```python
from build123d import *

# Parameters (mm, degrees)
F0_R     = 14.2875
F1_DEPTH = 14.2875
F2_R     = 6.35
F3_DEPTH = 44.45
F4_R     = 4.445
F5_DEPTH = 76.2


with BuildPart() as f1:
    # F0 (on Top) → F1 (new body, symmetric)
    with BuildSketch(Plane.XY):
        Circle(F0_R)
    extrude(amount=F1_DEPTH, both=True)

    # F2 (on face) → F3 (join)
    with BuildSketch(Plane(origin=(0, 0, -14.2875), x_dir=(1, 0, 0), z_dir=(0, 0, -1))):
        Circle(F2_R)
    extrude(amount=F3_DEPTH)

    # F4 (on Right) → F5 (join, symmetric)
    with BuildSketch(Plane.YZ):
        Circle(F4_R)
    extrude(amount=F5_DEPTH, both=True)

    # F6 (on Front) → F7 (revolve)
    with BuildSketch(Plane.XZ):
        with BuildLine():
            Line((-86.36, 0), (-66.04, 0))
            ThreePointArc((-66.04, 0), (-76.2, 10.16), (-86.36, 0))
        make_face()
    revolve(axis=Axis((-76.2, 0, 0), (1, 0, 0)))

    # F8 (on Front) → F9 (revolve)
    with BuildSketch(Plane.XZ):
        with BuildLine():
            Line((66.04, 0), (86.36, 0))
            ThreePointArc((86.36, 0), (76.2, 10.16), (66.04, 0))
        make_face()
    revolve(axis=Axis((76.2, 0, 0), (1, 0, 0)))


solid = f1.part
```
Model file for the job. Use its own axes, mm. A direction names the side the tool comes from. Give positions to 0.01 mm unless a question says otherwise; leave off trailing zeros. Write each loop counter-clockwise with the first axis right and the second up, starting at its lowest first coordinate (ties: lowest second). Pieces come first, ordered by that corner, then holes. Notation, with made-up numbers: (-35.5, 10.5) -> (16.5, 10.5) arc R21 ccw to (16.5, 33.5) -> close; hole circle Ø2 at (78, 78). An arc over 180 degrees is marked (long way). Use CSV: the item, a comma, the result in double quotes. Start each with the question number.
1) Cut at C-C on z = 0. List the corners of the cut face in (x, y) (1 decimal).
2) Cut at D-D on z = -28. List the corners of the cut face in (x, y).
3) Drill centre lines: L1, parallel to X at y = -0.25, z = -7; L2, parallel to X at y = -0.5, z = 6.5; L3, parallel to Z at x = 6, y = -12. Where is each one in solid material? Low to high.
4) Tool access for faces 4 (the cylindrical face through (-39.947, 2.051, -3.943)), 5 (the flat face through (0, 0, -58.738)): list every direction of +Z, -Z, +X, -X, +Y, -Y with a clear straight run to the whole face (end or side of a thin tool).
5) Two-plate mould, pull along X, no slides. Class faces 1 (the flat face through (6, -3, -14.288)), 2 (the cylindrical face through (-1.38, 6.2, -36.2)), 3 (the cylindrical face through (40.696, 2.051, -3.943)): released by +X, released by -X, zero draft, split by the parting line, or undercut.
6) Cut at A-A on x = 0. List the corners of the cut face in (y, z), plus the area to 3 significant figures.
7) Pin check, flat tips, straight feed: P1, Ø10, axis at y = -3, z = -1.5, coming from the +X side; P2, Ø6, axis at y = -8, z = -29, coming from the -X side; P3, Ø3, axis at x = -45, y = 2.5, coming from the -Z side; P4, Ø12, axis at y = -5, z = -44.5, coming from the +X side. Stop position of each tip, or through.
Final values:
1,outline,"(-67.1, -4.4) -> (-13.6, -4.4) arc R14.3 ccw to (13.6, -4.4) -> (67.1, -4.4) arc R10.2 ccw (long way) to (67.1, 4.4) -> (13.6, 4.4) arc R14.3 ccw to (-13.6, 4.4) -> (-67.1, 4.4) arc R10.2 ccw (long way) to start"
2,outline,"circle Ø12.7 at (0, 0)"
3,L1,"x = -83.56 to -68.84, -14.29 to 14.29, 68.84 to 83.56"
3,L2,"x = -83.99 to -68.41, -14.28 to 14.28, 68.41 to 83.99"
3,L3,"z = -14.29 to 14.29"
4,face 4,"none"
4,face 5,"-Z, +X, -X, +Y, -Y"
5,face 1,"zero draft"
5,face 2,"split by the parting line"
5,face 3,"undercut"
6,outline,"(-14.29, -14.29) -> (-6.35, -14.29) -> (-6.35, -58.74) -> (6.35, -58.74) -> (6.35, -14.29) -> (14.29, -14.29) -> (14.29, 14.29) -> (-14.29, 14.29) -> close"
6,area,"1,380 mm2"
7,P1,"stops at x = 86.36"
7,P2,"stops at x = -3.91"
7,P3,"stops at z = -4.33"
7,P4,"stops at x = 6.35"
